```python
from build123d import *

# Parameters (mm, degrees)
F2_S5_R     = 3.5814
F2_T6_DEPTH = 7


# Not quite as in the source:
# - a fillet or chamfer that OpenCascade refuses, or shapes differently, is made with other operations: its cross-section is extruded or revolved along the edge and cut away or added


with BuildPart() as f1:
    # F0 (on Front) → F1 (revolve)
    with BuildSketch(Plane.XZ):
        Polygon((0.889, -4.572), (1.651, -4.572), (1.9304, 0), (3.5814, 0), (3.5814, 0.889), (2.5273, 0.889), (2.3749, 4.064), (2.6289, 4.064), (2.032, 7.112), (1.27, 7.112), align=None)
    revolve(axis=Axis((0, 0, 1.778), (0, 0, 1)))

    # F2: chamfer of 1.27 on 1 edges, made by hand


with BuildPart() as f2_tool2:
    # F2_s3 → F2_t4 (revolve)
    with BuildSketch(Plane.XZ):
        Polygon((3.7973, 0.889), (2.4664101048, 2.1575394833), (2.5273, 0.889), align=None)
    revolve(axis=Axis((0, 0, 0.889), (0, 0, 1)))

    # F2_s5 → F2_t6 (intersect, symmetric)
    with BuildSketch(Plane.XY.offset(1.5)):
        Circle(F2_S5_R)
    extrude(amount=F2_T6_DEPTH, both=True, mode=Mode.INTERSECT)


with BuildPart() as f1_1:
    add(f1.part)

    # F2_t1: union F2_tool2
    add(f2_tool2.part)


solid = f1_1.part
```
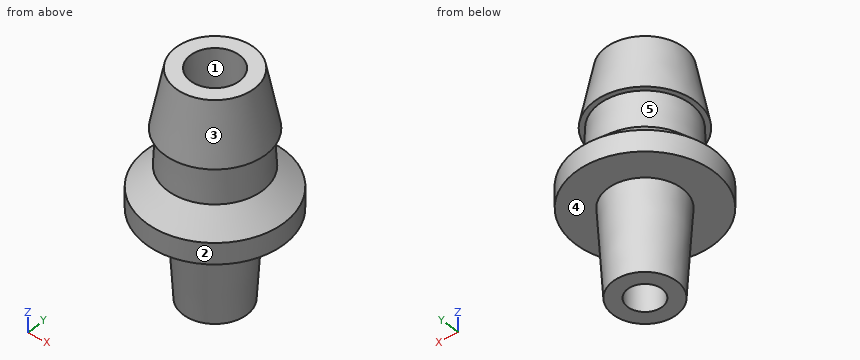
The model under review builds one solid part; all positions refer to its coordinate system, in mm. Face numbers are marked on the shaded views. A direction names the side the tool comes from. Coordinates: 2 decimals unless noted, no trailing zeros. Order: outer loops, then holes, each group sorted by start corner. A loop starts at its lowest first (then second) coordinate and runs counter-clockwise, first axis right, second up. Notation, with made-up numbers: (-34.75, 68) -> (-9.75, 68) arc R18 ccw to (-9.75, 85) -> close; hole circle Ø3 at (17, -39). An arc over 180 degrees is marked (long way). Answer in a Markdown table with one row per item. Add a question column.
Item 1: We need section C-C on z = 3.25. Write out the cut boundary in (x, y), plus the area to 3 significant figures.
Item 2: Mouldability with a two-part tool opening along Z and no side actions: class the marked faces 3, 4 and 5 as +Z half, -Z half, draft (parallel to the pull), parting line (faces both ways), or undercut.
Item 3: We need section A-A on x = 0. Write out the cut boundary in (y, z).
Item 4: Clearance check with a flat-ended pin moving along its axis: pin 1 (2 mm diameter, centred on x = -1, z = 2, fed in from -Y). State where the tip first meets the part, or that it passes through.
Item 5: We need section D-D on z = 5.5. Write out the cut boundary in (x, y), plus the area to 3 significant figures.
Item 6: Machinability: for the marked faces 1 and 2, which of the approach directions +Z, -Z, +X, -X, +Y, -Y give a long, thin tool a straight path to every point of the face, cutting with its end or side? Answer none if there is none.
Item 7: To check wall thickness, follow probe 1 along X at (y, z) = (0.75, 5.5); probe 2 along Y at (x, z) = (0, 2); probe 3 along X at (y, z) = (0, -2.5). State the ranges of each line that lie inside material, in increasing order.
Final values:
| question | item | result |
|---|---|---|
| 1 | outline | circle Ø4.83 at (0, 0); hole circle Ø2.29 at (0, 0) |
| 1 | area | 14.2 mm2 |
| 2 | face 3 | +Z half |
| 2 | face 4 | -Z half |
| 2 | face 5 | undercut |
| 3 | outline | (-3.58, 0) -> (-1.93, 0) -> (-1.65, -4.57) -> (-0.89, -4.57) -> (-1.27, 7.11) -> (-2.03, 7.11) -> (-2.63, 4.06) -> (-2.37, 4.06) -> (-2.47, 2.16) -> (-3.58, 1.09) -> close; (0.89, -4.57) -> (1.65, -4.57) -> (1.93, 0) -> (3.58, 0) -> (3.58, 1.09) -> (2.47, 2.16) -> (2.37, 4.06) -> (2.63, 4.06) -> (2.03, 7.11) -> (1.27, 7.11) -> close |
| 4 | pin 1 | stops at y = -3.53 |
| 5 | outline | circle Ø4.7 at (0, 0); hole circle Ø2.43 at (0, 0) |
| 5 | area | 12.7 mm2 |
| 6 | face 1 | +Z |
| 6 | face 2 | +Z, -Z |
| 7 | probe 1 | x = -2.22 to -0.96, 0.96 to 2.22 |
| 7 | probe 2 | y = -2.63 to -1.1, 1.1 to 2.63 |
| 7 | probe 3 | x = -1.78 to -0.96, 0.96 to 1.78 |
